Here's the drawing with two shaded views (mm, measured from the low corner). I have some questions. A direction names the side the tool comes from. Give positions to 0.01 mm unless a question says otherwise; leave off trailing zeros. Order: outer loops, then holes, each group sorted by start corner. A loop starts at its lowest first (then second) coordinate and runs counter-clockwise, first axis right, second up. Notation, with made-up numbers: (55, 76.5) - (62, 76.5) arc R11 cw to (62, 95.5) - close; hole circle Ø6 at (71, -35). An arc over 180 degrees is marked (long way). Use one line per item in the form item = value. Start each with the question number.
1) Suppose I cut it at D-D, the plane y = 8. Write out the boundary of the cut face in (x, z), and give its area (3 significant figures).
2) Suppose I cut it at B-B, the plane z = 26.15. Write out the boundary of the cut face in (x, y).
3) Suppose I cut it at A-A, the plane x = 52.3. Write out the boundary of the cut face in (y, z), and give its area (3 significant figures).
4) Please list where these lines run through material, in increasing order: probe 1 along X at (y, z) = (3.5, 10.65); probe 2 along Z at (x, y) = (5.65, 4.05); probe 3 along Z at (x, y) = (21.15, 3.6).
5) We'd pull the mould along X, two halves only. Please class the marked faces 5, 6 and 7: released by +X, released by -X, zero draft, split by the parting line, or undercut.
6) Which directions (+Z, -Z, +X, -X, +Y, -Y) give clear straight access to the entire face, cutting with the end or side of a thin tool? Please do the marked faces 1, 2, 3 and 4.
7) Suppose I cut it at C-C, the plane z = 36. Write out the boundary of the cut face in (x, y), and give its area (3 significant figures).
8) For pin 1 (4 mm diameter, centred on x = 13, y = 17, fed in from +Z); pin 2 (1.5 mm diameter, centred on x = 44, y = 31, fed in from +Z); pin 3 (2 mm diameter, centred on y = 14.5, z = 16, fed in from -X), each with a flat end and sliding along its axis, tell me the tip position at first contact or that it passes through.
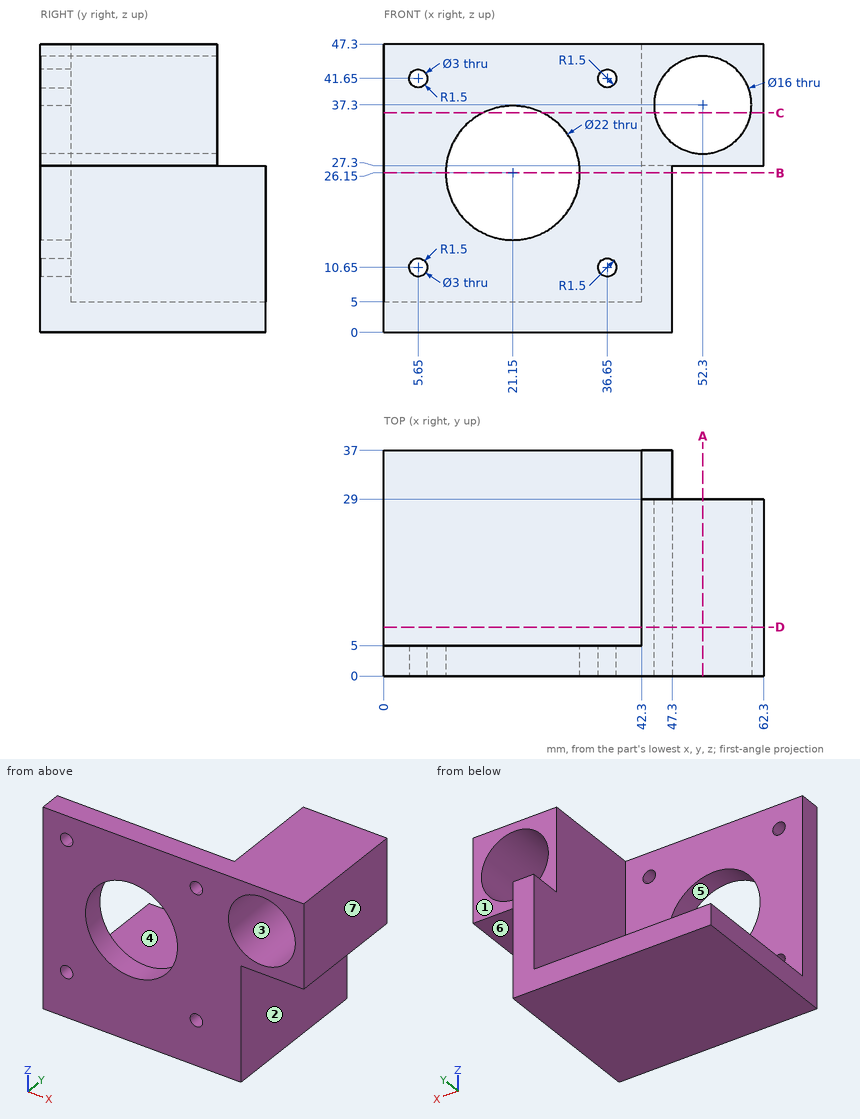
Result sheet:
q1.outline = (0, 0) - (47.3, 0) - (47.3, 27.3) - (62.3, 27.3) - (62.3, 47.3) - (42.3, 47.3) - (42.3, 5) - (0, 5) - close; hole circle Ø16 at (52.3, 37.3)
q1.area = 547 mm²
q2.outline = (0, 0) - (10.15, 0) - (10.15, 5) - (0, 5) - close; (32.15, 0) - (47.3, 0) - (47.3, 37) - (42.3, 37) - (42.3, 5) - (32.15, 5) - close
q3.outline = (0, 27.3) - (29, 27.3) - (29, 29.3) - (0, 29.3) - close; (0, 45.3) - (29, 45.3) - (29, 47.3) - (0, 47.3) - close
q3.area = 116 mm²
q4.probe_1 = 0 to 4.15, 7.15 to 35.15, 38.15 to 47.3
q4.probe_2 = 0 to 9.15, 12.15 to 40.15, 43.15 to 47.3
q4.probe_3 = 0 to 15.15, 37.15 to 47.3
q5.face_5 = undercut
q5.face_6 = zero draft
q5.face_7 = released by +X
q6.face_1 = +Z, +X, -X, +Y
q6.face_2 = -Z, +X, +Y, -Y
q6.face_3 = +Y, -Y
q6.face_4 = +Z, -X, +Y
q7.outline = (0, 0) - (16.25, 0) - (16.25, 5) - (0, 5) - close; (26.05, 0) - (44.41, 0) - (44.41, 29) - (42.3, 29) - (42.3, 5) - (26.05, 5) - close; (60.19, 0) - (62.3, 0) - (62.3, 29) - (60.19, 29) - close
q7.area = 285 mm²
q8.pin_1 = 5
q8.pin_2 = 27.3
q8.pin_3 = 42.3
